Could you check a few things on this model? Use its own coordinates, in mm. Face numbers are marked on the shaded views. Give positions to 0.01 mm unless a question says otherwise; leave off trailing zeros. Loops run counter-clockwise (first coordinate to the right, second up) from the corner with the lowest first, then second, coordinate; pieces in that order, holes last. Notation, with made-up numbers: M 80,29.5 L 86,29.5 A14 cw 86,43.5 Z; hole C -17.5,-1.75 d11. An arc over 180 degrees is marked long. Use a Markdown table: item, result. Add a question column.
1) Suppose I cut it at B-B on x = 25.4. List the corners of the cut face in (y, z) for me, and give its area (3 significant figures).
2) We'd pull the mould along Y, two halves only. Please class the marked faces 1 and 2: +Y half, -Y half, draft (parallel to the pull), parting line (faces both ways), or undercut.
3) If I drill on line 1 along Z through (x, y) = (0, 1); line 2 along Z through (x, y) = (16, 0.6); line 3 along Z through (x, y) = (25.4, 1.15), over which ranges is the centre line in solid material (lowest first)? Write a range as [from, to].
4) Suppose I cut it at A-A on y = 0.9. List the corners of the cut face in (x, z) for me.
5) Suppose I cut it at D-D on x = 19. List the corners of the cut face in (y, z) for me, and give its area (3 significant figures).
6) Suppose I cut it at C-C on z = 20. List the corners of the cut face in (x, y) for me.
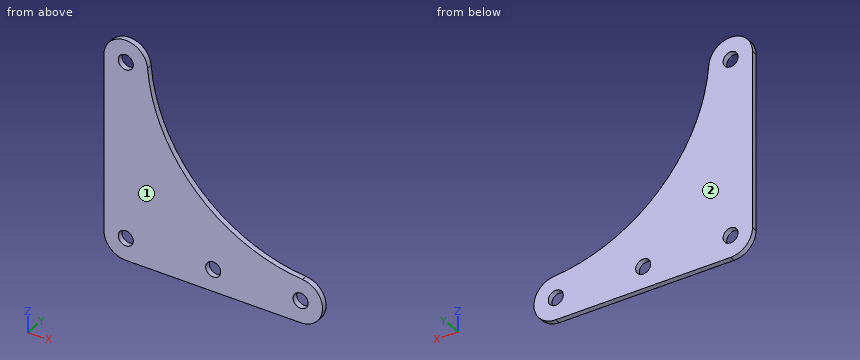
Autodesk Inventor part; units mm, degrees
ref_plane "YZ Plane" through (0, 0, 0) normal (1, 0, 0) x (0, 1, 0)
ref_plane "XZ Plane" through (0, 0, 0) normal (0, 1, 0) x (-1, 0, 0)
ref_plane "XY Plane" through (0, 0, 0) normal (0, 0, 1) x (1, 0, 0)
sketch "main" plane through (0, 0, 0) normal (0, 0, 1) x (1, 0, 0)
  circle A0 centre (27.8145, 23.5161) radius 2.1844
  circle A1 centre (27.8145, -27.2839) radius 2.1844
  circle A2 centre (-22.9855, -27.2839) radius 2.1844
  arc A3 (-23.5053, -20.9552) -> (-22.9855, -33.6339) centre (-22.9855, -27.2839) ccw
  arc A4 (27.8145, -33.6339) -> (34.1645, -27.2839) centre (27.8145, -27.2839) ccw
  arc A5 (34.1645, 23.5161) -> (21.4858, 24.0358) centre (27.8145, 23.5161) ccw
  line L0 (34.1645, 23.5161) -> (34.1645, -27.2839)
  line L1 (27.8145, -33.6339) -> (-22.9855, -33.6339)
  arc A6 (-23.5053, -20.9552) -> (21.4858, 24.0358) centre (-27.5308, 28.0614) ccw
  point P0 (11.2944, -10.7639)
sketch "Sketch1" plane through (0, 0, 0) normal (0, 1, 0) x (-1, 0, 0)
  circle A0 centre (-25.4, 0) radius 2.1844
  circle A1 centre (0, 50.8) radius 2.1844
  circle A2 centre (0, 0) radius 2.1844
  circle A3 centre (-50.8, 0) radius 2.1844
  arc A4 (-51.3197, 6.3287) -> (-50.8, -6.35) centre (-50.8, 0) ccw
  arc A5 (0, -6.35) -> (6.35, 0) centre (0, 0) ccw
  arc A6 (6.35, 50.8) -> (-6.3287, 51.3197) centre (0, 50.8) ccw
  line L0 (6.35, 50.8) -> (6.35, 0)
  line L1 (0, -6.35) -> (-50.8, -6.35)
  arc A7 (-51.3197, 6.3287) -> (-6.3287, 51.3197) centre (-55.3453, 55.3453) ccw
  dimension "d2" = 4.3688
extrude "Extrusion1" add sketch "Sketch1" along normal blind 1.5875
equation "\"BendRadius\" = Thickness"
equation "\"BendReliefWidth\" = Thickness"
equation "\"BendReliefDepth\" = 0.5 * Thickness"
equation "\"CornerReliefSize\" = 4 * Thickness"
equation "\"MinimumRemnant\" = 2 * Thickness"
equation "\"TransitionRadius\" = BendRadius"
equation "\"JacobiRadiusSize\" = BendRadius"
equation "\"GapSize\" = Thickness"
properties part number "Arm Triangle Gusset" material "Acetal Resin, White"
Answer block:
| question | item | result |
|---|---|---|
| 1 | outline | M 0,-6.35 L 1.59,-6.35 L 1.59,-2.18 L 0,-2.18 Z; M 0,2.18 L 1.59,2.18 L 1.59,16.33 L 0,16.33 Z |
| 1 | area | 29.1 mm^2 |
| 2 | face 1 | -Y half |
| 2 | face 2 | +Y half |
| 3 | line 1 | z = [-6.35, -2.18], [2.18, 48.62], [52.98, 57.15] |
| 3 | line 2 | z = [-6.35, 25.84] |
| 3 | line 3 | z = [-6.35, -2.18], [2.18, 16.33] |
| 4 | outline | M -6.35,0 A6.35 ccw 0,-6.35 L 50.8,-6.35 A6.35 ccw 51.32,6.33 A49.18 cw 6.33,51.32 A6.35 ccw -6.35,50.8 Z; hole C 0,0 d4.37; hole C 0,50.8 d4.37; hole C 25.4,0 d4.37; hole C 50.8,0 d4.37 |
| 5 | outline | M 0,-6.35 L 1.59,-6.35 L 1.59,22.21 L 0,22.21 Z |
| 5 | area | 45.3 mm^2 |
| 6 | outline | M -6.35,0 L 21.15,0 L 21.15,1.59 L -6.35,1.59 Z |
